Source: CAD feature listing. Evaluate the final solid. Frame: model axes, mm. Coordinates: 2 decimals unless noted, no trailing zeros. Write each loop counter-clockwise with the first axis right and the second up, starting at its lowest first coordinate (ties: lowest second). Pieces come first, ordered by that corner, then holes. Notation, with made-up numbers: M -27,85.25 L 28,85.25 A26 cw 28,124.25 Z; hole C 9,-15 d8. An arc over 180 degrees is marked long. One line per item, written item: value. Start each with the question number.
Item 1: Cut plane B-B, the plane y = 5.4. Output: boundary loops of the cut face in (x, z), then the cut area to 3 significant figures.
Item 2: Ray query, L1, parallel to X at y = 1.45, z = 0.1; L2, parallel to X at y = 4.85, z = 0.2; L3, parallel to Y at x = 6.5, z = 0.1. Return the intervals inside material, ascending. Write a range as from..to.
Item 3: Cut plane C-C, the plane y = 4.6. Output: boundary loops of the cut face in (x, z), then the cut area to 3 significant figures.
Item 4: Cut plane A-A, the plane y = 2.25. Output: boundary loops of the cut face in (x, z), then the cut area to 3 significant figures.
```python
from build123d import *

# Parameters (mm, degrees)
RESSALTO_EXTRUS_O1_DEPTH = 0.27
FILETE5_R                = 0.1


with BuildPart() as part:
    # Esboço1 → Ressalto-extrusão1 (new body)
    with BuildSketch(Plane.XY):
        Polygon((0, 0), (0, 3.270833333), (6.53125, 4.729166667), (6.53125, 6), (7.294533781, 6), (7.294533781, 4.255670993), (6.629245544, 4.107740982), (0.25, 2.689285325), (0.25, 0), align=None)
    extrude(amount=RESSALTO_EXTRUS_O1_DEPTH)

    # Filete5
    filete5_edges = [part.edges().sort_by_distance(p)[0] for p in [
        (3.772266891, 3.472478159, 0.27),
        (3.772266891, 3.472478159, 0),
        (0.25, 1.344642663, 0),
        (0, 0, 0.135),
        (0, 3.270833333, 0.135),
        (7.294533781, 4.255670993, 0.135),
        (0.25, 2.689285325, 0.135),
        (0, 1.635416667, 0.27),
        (0.25, 1.344642663, 0.27),
        (0, 1.635416667, 0),
    ]]
    fillet(filete5_edges, radius=FILETE5_R)


solid = part.part
```
From the geometry:
1. outline: M 6.53,0 L 7.29,0 L 7.29,0.27 L 6.53,0.27 Z
1. area: 0.206 mm²
2. L1: x = 0..0.25
2. L2: x = 6.53..7.29
2. L3: y = 4.08..4.72
3. outline: M 5.95,0 L 7.29,0 L 7.29,0.27 L 5.95,0.27 Z
3. area: 0.362 mm²
4. outline: M 0,0.1 A0.1 ccw 0.1,0 L 0.15,0 A0.1 ccw 0.25,0.1 L 0.25,0.17 A0.1 ccw 0.15,0.27 L 0.1,0.27 A0.1 ccw 0,0.17 Z
4. area: 0.0589 mm²
